Design review of the part built by this model. Coordinates are the model's own, in mm. A direction names the side the tool comes from. Give positions to 0.01 mm unless a question says otherwise; leave off trailing zeros. Loops run counter-clockwise (first coordinate to the right, second up) from the corner with the lowest first, then second, coordinate; pieces in that order, holes last. Notation, with made-up numbers: (49.5, -39.5) -> (96.5, -39.5) arc R26 cw to (96.5, -21.5) -> close; hole circle Ø11 at (16.25, 30). An arc over 180 degrees is marked (long way). Use a Markdown table: item, result. Add a question column.
1. Add section D-D (x = -7.5). State the section outline as (y, z) points.
2. Add section B-B (y = -0.1). Count the separate pieces of the cut face and the enclosed holes in it, and give its area (3 significant figures).
3. For pin 1 Ø2 at (x, z) = (28, -41.5) entering from -Y, flat-tipped, find the tip position at first contact; note if it passes through.
4. To check wall thickness, follow line 1 (Z direction, x = -28, y = -0.15); line 2 (X direction, y = 0.45, z = 41.5); line 3 (X direction, y = -0.3, z = -41.5). State the ranges of each line that lie inside material, in increasing order.
5. Add section C-C (z = 24.5). State the section outline as (x, y) points (3 decimals), and give its area (3 significant figures).
6. For faces 1 (the cylindrical face through (-30.9, 0.01, -0.27)), 2 (the cylindrical face through (23.9, 0, -40.2)), 3 (the cylindrical face through (30.93, 0.01, -0.3)), list the 3-axis set-ups (+Z, -Z, +X, -X, +Y, -Y) from which the entire face can be reached by the end or side of a thin tool; tool diameter is ignored.
7. Draft analysis for pull direction X (two halves, no side actions). For faces 4 (the cylindrical face through (-30.9, 0.01, 44.43)), 5 (the cylindrical face through (30.9, 0.01, -44.43)), 6 (the cylindrical face through (27.33, -0.01, 43.117)), 7 (the cylindrical face through (-23.9, 0, -40.2)), state which applies: pulls with the +X half, pulls with the -X half, needs draft (parallel to the pull), parting line crosses it, or undercut.
8. Add section A-A (z = 41.5). State the section outline as (x, y) points, and give its area (3 significant figures).
```python
from build123d import *

# Parameters (mm, degrees)
SKETCH1_R           = 1.75
BOSS_EXTRUDE1_DEPTH = 0.75


with BuildPart() as part:
    # Sketch1 → Boss-Extrude1 (new, symmetric)
    with BuildSketch(Plane(origin=(0, 0, 0), x_dir=(1, 0, 0), z_dir=(0, 1, 0))):
        with BuildLine():
            Line((29.5, -0.3), (22.925, -0.3))
            ThreePointArc((22.925, -0.3), (21.510786438, -0.885786438), (20.925, -2.3))
            Line((20.925, -2.3), (20.925, -31.3))
            ThreePointArc((20.925, -31.3), (21.510786438, -32.714213562), (22.925, -33.3))
            Line((22.925, -33.3), (29.5, -33.3))
            ThreePointArc((29.5, -33.3), (30.914213562, -33.885786438), (31.5, -35.3))
            Line((31.5, -35.3), (31.5, -43))
            ThreePointArc((31.5, -43), (30.914213562, -44.414213562), (29.5, -45))
            Line((29.5, -45), (-29.5, -45))
            ThreePointArc((-29.5, -45), (-30.914213562, -44.414213562), (-31.5, -43))
            Line((-31.5, -43), (-31.5, -35.3))
            ThreePointArc((-31.5, -35.3), (-30.914213562, -33.885786438), (-29.5, -33.3))
            Line((-29.5, -33.3), (-22.925, -33.3))
            ThreePointArc((-22.925, -33.3), (-21.510786438, -32.714213562), (-20.925, -31.3))
            Line((-20.925, -31.3), (-20.925, -2.3))
            ThreePointArc((-20.925, -2.3), (-21.510786438, -0.885786438), (-22.925, -0.3))
            Line((-22.925, -0.3), (-29.5, -0.3))
            ThreePointArc((-29.5, -0.3), (-30.914213562, 0.285786438), (-31.5, 1.7))
            Line((-31.5, 1.7), (-31.5, 43))
            ThreePointArc((-31.5, 43), (-30.914213562, 44.414213562), (-29.5, 45))
            Line((-29.5, 45), (-26.5, 45))
            ThreePointArc((-26.5, 45), (-25.085786438, 44.414213562), (-24.5, 43))
            Line((-24.5, 43), (-24.5, 41.631016383))
            ThreePointArc((-24.5, 41.631016383), (-23.914213562, 40.216802821), (-22.5, 39.631016383))
            Line((-22.5, 39.631016383), (22.5, 39.631016383))
            ThreePointArc((22.5, 39.631016383), (23.914213562, 40.216802821), (24.5, 41.631016383))
            Line((24.5, 41.631016383), (24.5, 43))
            ThreePointArc((24.5, 43), (25.085786438, 44.414213562), (26.5, 45))
            Line((26.5, 45), (29.5, 45))
            ThreePointArc((29.5, 45), (30.914213562, 44.414213562), (31.5, 43))
            Line((31.5, 43), (31.5, 1.7))
            ThreePointArc((31.5, 1.7), (30.914213562, 0.285786438), (29.5, -0.3))
        make_face()
        with Locations(Location((27.996318987, 41.5, 0), (0, 0, 270))):
            Circle(SKETCH1_R, mode=Mode.SUBTRACT)
        with Locations(Location((-27.996318987, 41.5, 0), (0, 0, 90))):
            Circle(SKETCH1_R, mode=Mode.SUBTRACT)
        with Locations(Location((28, -41.5, 0), (0, 0, 270))):
            Circle(SKETCH1_R, mode=Mode.SUBTRACT)
        with Locations(Location((-28, -41.5, 0), (0, 0, 90))):
            Circle(SKETCH1_R, mode=Mode.SUBTRACT)
    extrude(amount=BOSS_EXTRUDE1_DEPTH, both=True)


solid = part.part
```
Taken from the geometry:
| question | item | result |
|---|---|---|
| 1 | outline | (-0.75, -39.63) -> (0.75, -39.63) -> (0.75, 45) -> (-0.75, 45) -> close |
| 2 | separate pieces | 1 |
| 2 | enclosed holes | 4 |
| 2 | area | 4,670 mm^2 |
| 3 | pin 1 | passes through |
| 4 | line 1 | z = -45 to -43.25, -39.75 to 0.3, 33.3 to 39.75, 43.25 to 45 |
| 4 | line 2 | x = -31.5 to -29.75, -26.25 to 26.25, 29.75 to 31.5 |
| 4 | line 3 | x = -31.5 to -29.75, -26.25 to -24.5, 24.5 to 26.25, 29.75 to 31.5 |
| 5 | outline | (-20.925, -0.75) -> (20.925, -0.75) -> (20.925, 0.75) -> (-20.925, 0.75) -> close |
| 5 | area | 62.8 mm^2 |
| 6 | face 1 | -X, +Y, -Y |
| 6 | face 2 | -Z, +Y, -Y |
| 6 | face 3 | +X, +Y, -Y |
| 7 | face 4 | pulls with the -X half |
| 7 | face 5 | pulls with the +X half |
| 7 | face 6 | undercut |
| 7 | face 7 | undercut |
| 8 | outline | (-31.5, -0.75) -> (-29.75, -0.75) -> (-29.75, 0.75) -> (-31.5, 0.75) -> close; (-26.25, -0.75) -> (26.25, -0.75) -> (26.25, 0.75) -> (-26.25, 0.75) -> close; (29.75, -0.75) -> (31.5, -0.75) -> (31.5, 0.75) -> (29.75, 0.75) -> close |
| 8 | area | 84.0 mm^2 |
